Part model, mm, in its own coordinate system. A direction names the side the tool comes from. Round coordinates to 2 decimals unless told otherwise and drop trailing zeros. Order: outer loops, then holes, each group sorted by start corner. A loop starts at its lowest first (then second) coordinate and runs counter-clockwise, first axis right, second up. Notation, with made-up numbers: (-39.75, 8) - (-21.75, 8) arc R24 ccw to (-21.75, 27) - close; hole circle Ø9 at (-29, 54). An arc over 180 degrees is marked (long way). Return JSON: item names as keys, results as strings. Group by question number.
Item 1: Drop flat-ended pins along their axis: pin 1 (0.9 mm diameter, centred on y = 1.5, z = 8, fed in from -X); pin 2 (12 mm diameter, centred on x = -11.5, z = 35.5, fed in from +Y); pin 3 (1.8 mm diameter, centred on x = -13.175, z = 12.5, fed in from +Y); pin 4 (0.9 mm diameter, centred on y = 2, z = 8, fed in from +X). Give the stop position or say it passes through.
Item 2: Saw through at C-C on y = 1.95. State how many separate pieces and enclosed holes the cut face has, and give its area (3 significant figures).
Item 3: Saw through at B-B on x = -16. List the corners of the cut face in (y, z).
Item 4: Saw through at A-A on z = 31. List the corners of the cut face in (x, y) (3 decimals).
Item 5: Two-plate mould, pull along X, no slides. Class faces 5 (the face through (2, 1, 40)), 6 (the face through (3, 1, 16)), 7 (the face through (-7.175, 1, 26)): released by +X, released by -X, zero draft, split by the parting line, or undercut.
Item 6: Tool access for faces 1 (the face through (-28, 1, 12)), 2 (the face through (-13, 1, 15)), 3 (the face through (1, 1, 33)), 4 (the face through (-28, 1, 19)): list every direction of +Z, -Z, +X, -X, +Y, -Y with a clear straight run to the whole face (end or side of a thin tool).
Item 7: Probe probe 1 along Z at (x, y) = (-27, 2.85); probe 2 along X at (y, z) = (2.9, 35) (3 decimals); probe 3 along X at (y, z) = (2.2, 32.5) (3 decimals). List the from-to ranges inside material, lowest first.
Autodesk Inventor part; units mm, degrees
ref_plane "YZ Plane" through (0, 0, 0) normal (1, 0, 0) x (0, 1, 0)
ref_plane "XZ Plane" through (0, 0, 0) normal (0, 1, 0) x (-1, 0, 0)
ref_plane "XY Plane" through (0, 0, 0) normal (0, 0, 1) x (1, 0, 0)
sketch "Boceto1" plane through (0, 0, 0) normal (0, 1, 0) x (-1, 0, 0)
  line L0 (0, 0) -> (26.35, 0)
  line L1 (26.35, 10) -> (0, 10)
  line L2 (26.35, 10) -> (29.35, 10)
  line L3 (29.35, 10) -> (29.35, 0)
  line L4 (29.35, 0) -> (26.35, 0)
  line L5 (0, 10) -> (-3, 10)
  line L6 (-3, 10) -> (-3, 0)
  line L7 (-3, 0) -> (0, 0)
extrude "Extrusión1" add sketch "Boceto1" along normal blind 3
sketch "Boceto2" plane through (0, 0, 0) normal (0, -1, 0) x (1, 0, 0)
  line L0 (-26.35, 10) -> (-26.35, 40)
  line L1 (-26.35, 47) -> (0, 47)
  line L2 (0, 40) -> (0, 10)
  line L3 (-26.35, 10) -> (0, 10)
  line L4 (-13.175, 15) -> (-7.175, 15)
  line L5 (-7.175, 15) -> (-7.175, 38)
  line L6 (-7.175, 38) -> (-19.175, 38)
  line L7 (-19.175, 38) -> (-19.175, 15)
  line L8 (-19.175, 15) -> (-13.175, 15)
  circle A0 centre (-13.175, 40.5) radius 1.5
  circle A1 centre (-13.175, 12.5) radius 1.5
  line L9 (-26.35, 47) -> (-29.35, 47)
  line L10 (-29.35, 47) -> (-29.35, 40)
  line L11 (-29.35, 40) -> (-26.35, 40)
  line L12 (0, 47) -> (3, 47)
  line L13 (3, 47) -> (3, 40)
  line L14 (3, 40) -> (0, 40)
  point P0 (0, 0)
  dimension "d19" = 7
  dimension "d20" = 3
extrude "Extrusión2" add sketch "Boceto2" against normal blind 3
sketch "Boceto3" plane through (0, 0, 0) normal (0, -1, 0) x (1, 0, 0)
  line L0 (0, 33) -> (3, 33)
  line L1 (3, 33) -> (3, 26)
  line L2 (3, 26) -> (0, 26)
  line L3 (0, 26) -> (0, 33)
  line L4 (-26.35, 33) -> (-29.35, 33)
  line L5 (-29.35, 33) -> (-29.35, 26)
  line L6 (-29.35, 26) -> (-26.35, 26)
  line L7 (-26.35, 26) -> (-26.35, 33)
  line L8 (-26.35, 19) -> (-29.35, 19)
  line L9 (-29.35, 19) -> (-29.35, 12)
  line L10 (-29.35, 12) -> (-26.35, 12)
  line L11 (-26.35, 12) -> (-26.35, 19)
  line L12 (0, 19) -> (3, 19)
  line L13 (3, 19) -> (3, 12)
  line L14 (3, 12) -> (0, 12)
  line L15 (0, 12) -> (0, 19)
  point P0 (0, 0)
  point P1 (0, 40)
extrude "Extrusión3" add sketch "Boceto3" against normal blind 3
sketch "Boceto4" plane through (0, 0, 0) normal (0, -1, 0) x (1, 0, 0)
  line L0 (-13.175, 5.5) -> (-26.35, 5.5)
  line L1 (-26.35, 5.5) -> (-29.35, 5.5)
  line L2 (-29.35, 0) -> (-29.35, 10)
  line L3 (-13.175, 5.5) -> (3, 5.5)
  line L4 (3, 10) -> (3, 0)
  line L5 (3, 0) -> (-29.35, 0)
  line L6 (3, 5.5) -> (3, 0)
  line L7 (3, 0) -> (-29.35, 0)
  line L8 (-29.35, 0) -> (-29.35, 5.5)
  point P0 (0, 0)
  point P1 (-13.175, 12.5)
  point P2 (-26.35, 10)
extrude "Extrusión4" cut sketch "Boceto4" against normal blind 3
sketch "Boceto5" plane through (0, 0, 0) normal (0, -1, 0) x (1, 0, 0)
  line L0 (-26.35, 10) -> (-26.35, 12)
  line L1 (-26.35, 10) -> (-26.35, 5.5)
  line L2 (-26.35, 5.5) -> (-29.35, 5.5)
  line L3 (-29.35, 10) -> (-26.35, 10)
  line L4 (-29.35, 5.5) -> (-29.35, 10)
  line L5 (-29.35, 10) -> (-26.35, 10)
  line L6 (0, 10) -> (3, 10)
  line L7 (0, 10) -> (3, 10)
  line L8 (3, 10) -> (3, 5.5)
  line L9 (3, 10) -> (3, 5.5)
  line L10 (3, 5.5) -> (0, 5.5)
  line L11 (0, 10) -> (0, 5.5)
  point P0 (0, 0)
extrude "Extrusión5" cut sketch "Boceto5" against normal blind 3
properties part number "muñeca1"
Filled in:
{
 "1": {"pin 1": "stops at x = -26.35", "pin 2": "stops at y = 3", "pin 3": "passes through", "pin 4": "stops at x = 0"},
 "2": {"separate pieces": "1", "enclosed holes": "3", "area": "929 mm^2"},
 "3": {"outline": "(0, 5.5) - (3, 5.5) - (3, 15) - (0, 15) - close; (0, 38) - (3, 38) - (3, 47) - (0, 47) - close"},
 "4": {"outline": "(-29.35, 0) - (-19.175, 0) - (-19.175, 3) - (-29.35, 3) - close; (-7.175, 0) - (3, 0) - (3, 3) - (-7.175, 3) - close"},
 "5": {"face 5": "zero draft", "face 6": "released by +X", "face 7": "undercut"},
 "6": {"face 1": "-Z, -X, +Y, -Y", "face 2": "+Y, -Y", "face 3": "+X, +Y, -Y", "face 4": "-X, +Y, -Y"},
 "7": {"probe 1": "z = 12 to 19, 26 to 33, 40 to 47", "probe 2": "x = -26.35 to -19.175, -7.175 to 0", "probe 3": "x = -29.35 to -19.175, -7.175 to 3"}
}
